Autodesk Fusion 360 part; units mm, degrees
sketch "Sketch1" plane through (0, 0, 0) normal (0, 1, 0) x (1, 0, 0)
  line L0 (0, 0) -> (0, -12.7)
  line L1 (0, -12.7) -> (38.1, -12.7)
  line L2 (38.1, -12.7) -> (38.1, -38.1)
  line L3 (0, 0) -> (88.9, 0)
  line L4 (88.9, 0) -> (88.9, -38.1)
  arc A0 (38.1, -38.1) -> (88.9, -38.1) centre (63.5, -38.1) ccw
  circle A1 centre (63.5, -38.1) radius 12.7
extrude "Extrude1" add sketch "Sketch1" along normal mid plane 50.8
sketch "Sketch2" plane through (88.9, 0, 0) normal (1, 0, 0) x (0, 1, 0)
  line L0 (-25.4, 0) -> (25.4, 0)
  line L1 (25.4, 0) -> (25.4, 38.1)
  line L2 (25.4, 38.1) -> (-25.4, 38.1)
  line L3 (-25.4, 38.1) -> (-25.4, 0)
  line L4 (-12.7, 67.4271) -> (-12.7, 12.7)
  line L5 (-12.7, 12.7) -> (12.7, 12.7)
  line L6 (12.7, 12.7) -> (12.7, 67.4271)
  line L7 (-12.7, 63.5) -> (12.7, 63.5)
  dimension "d3" = 12.7
  dimension "d4" = 12.7
  dimension "d5" = 12.7
extrude "Extrude2" cut sketch "Sketch2" against normal blind 50.8 contours L2 L4 L6 L7 | L2 L4 L5 L6
sketch "Sketch3" plane through (0, 0, 0) normal (-1, 0, 0) x (0, -1, 0)
  line L0 (25.4, 12.7) -> (-25.4, 12.7)
  line L1 (-25.4, 12.7) -> (-25.4, 0)
  line L2 (-25.4, 0) -> (25.4, 0)
  line L3 (25.4, 0) -> (25.4, 12.7)
fillet "Fillet1" radius 25.4 1 edges at (0, -25.4, 6.35)
fillet "Fillet2" radius 25.4 1 edges at (0, 25.4, 6.35)
Could you check a few things on this model? Use its own coordinates, in mm. A direction names the side the tool comes from. Give positions to 0.01 mm unless a question says otherwise; leave off trailing zeros. Order: outer loops, then holes, each group sorted by start corner. A loop starts at its lowest first (then second) coordinate and runs counter-clockwise, first axis right, second up.
1. Suppose I cut it at C-C (y = 20.5). Write out the boundary of the cut face in (x, z), plus the area to 3 significant figures.
Answers below:
outline: (10.4, 0) - (88.9, 0) - (88.9, 38.1) arc R25.4 ccw to (38.1, 38.1) - (38.1, 12.7) - (10.4, 12.7) - close; hole circle Ø25.4 at (63.5, 38.1)
area: 2,790 mm2
2. Suppose I cut it at B-B (z = 19.5). Write out the boundary of the cut face in (x, y), plus the area to 3 significant figures.
Answers below:
outline: (38.1, -25.4) - (88.9, -25.4) - (88.9, -12.7) - (38.1, -12.7) - close; (38.1, 12.7) - (88.9, 12.7) - (88.9, 25.4) - (38.1, 25.4) - close
area: 1,290 mm2
3. Suppose I cut it at A-A (x = 63.5). Write out the boundary of the cut face in (y, z), plus the area to 3 significant figures.
Answers below:
outline: (-25.4, 0) - (25.4, 0) - (25.4, 25.4) - (12.7, 25.4) - (12.7, 12.7) - (-12.7, 12.7) - (-12.7, 25.4) - (-25.4, 25.4) - close; (-25.4, 50.8) - (-12.7, 50.8) - (-12.7, 63.5) - (-25.4, 63.5) - close; (12.7, 50.8) - (25.4, 50.8) - (25.4, 63.5) - (12.7, 63.5) - close
area: 1,290 mm2
4. Which directions (+Z, -Z, +X, -X, +Y, -Y) give clear straight access to the entire face, cutting with the end or side of a thin tool? Please do faces 5 (the cylindrical face through (7.24, -17.76, 6.44)), 6 (the flat face through (38.1, 19, 25)).
Answers below:
face 5: +Z, -Z, -X, -Y
face 6: +Z, -X, +Y, -Y
5. I need wall thicknesses on L1, parallel to Y at x = 53.5, z = 18; L2, parallel to X at y = 22, z = 38; L3, parallel to Z at x = 63.5, y = 17. Which ranges of each line are inside material? Lowest first, please.
Answers below:
L1: y = -25.4 to -12.7, 12.7 to 25.4
L2: x = 38.1 to 50.8, 76.2 to 88.9
L3: z = 0 to 25.4, 50.8 to 63.5
6. For pin 1 (4 mm diameter, centred on y = 20.5, z = 27.5, fed in from -X); pin 2 (2 mm diameter, centred on x = 11, y = 10.5, fed in from +Z); pin 3 (20.5 mm diameter, centred on x = 63.5, z = 38.1, fed in from +Y); pin 4 (3 mm diameter, centred on y = 10.5, z = 13.5, fed in from +X), each with a flat end and sliding along its axis, tell me the tip position at first contact or that it passes through.
Answers below:
pin 1: stops at x = 38.1
pin 2: stops at z = 12.7
pin 3: passes through
pin 4: stops at x = 88.9
7. Thinking about a two-plate mould opening in Y: for faces 1 (the flat face through (64, 25.4, 24)), 2 (the cylindrical face through (75.614, 18.961, 41.915)), 3 (the flat face through (64, -12.7, 22)), 4 (the flat face through (70, 12.7, 26)), which applies, +Y half, -Y half, draft (parallel to the pull), parting line (faces both ways), or undercut?
Answers below:
face 1: +Y half
face 2: draft
face 3: undercut
face 4: undercut
8. Suppose I cut it at D-D (z = 46). Write out the boundary of the cut face in (x, y).
Answers below:
outline: (39.36, -25.4) - (53.56, -25.4) - (53.56, -12.7) - (39.36, -12.7) - close; (39.36, 12.7) - (53.56, 12.7) - (53.56, 25.4) - (39.36, 25.4) - close; (73.44, -25.4) - (87.64, -25.4) - (87.64, -12.7) - (73.44, -12.7) - close; (73.44, 12.7) - (87.64, 12.7) - (87.64, 25.4) - (73.44, 25.4) - close
